Source: three-view drawing plus pictorial views. Frame: mm from the lowest corner of the part. A direction names the side the tool comes from. Give positions to 0.01 mm unless a question says otherwise; leave off trailing zeros. Order: outer loops, then holes, each group sorted by start corner. A loop starts at its lowest first (then second) coordinate and runs counter-clockwise, first axis right, second up. Notation, with made-up numbers: (-25.5, -15) -> (-3.5, -15) arc R36 cw to (-3.5, 22) -> close; hole circle Ø9 at (-26, 45.25). An arc over 180 degrees is marked (long way). Answer in a Markdown table with one row per item.
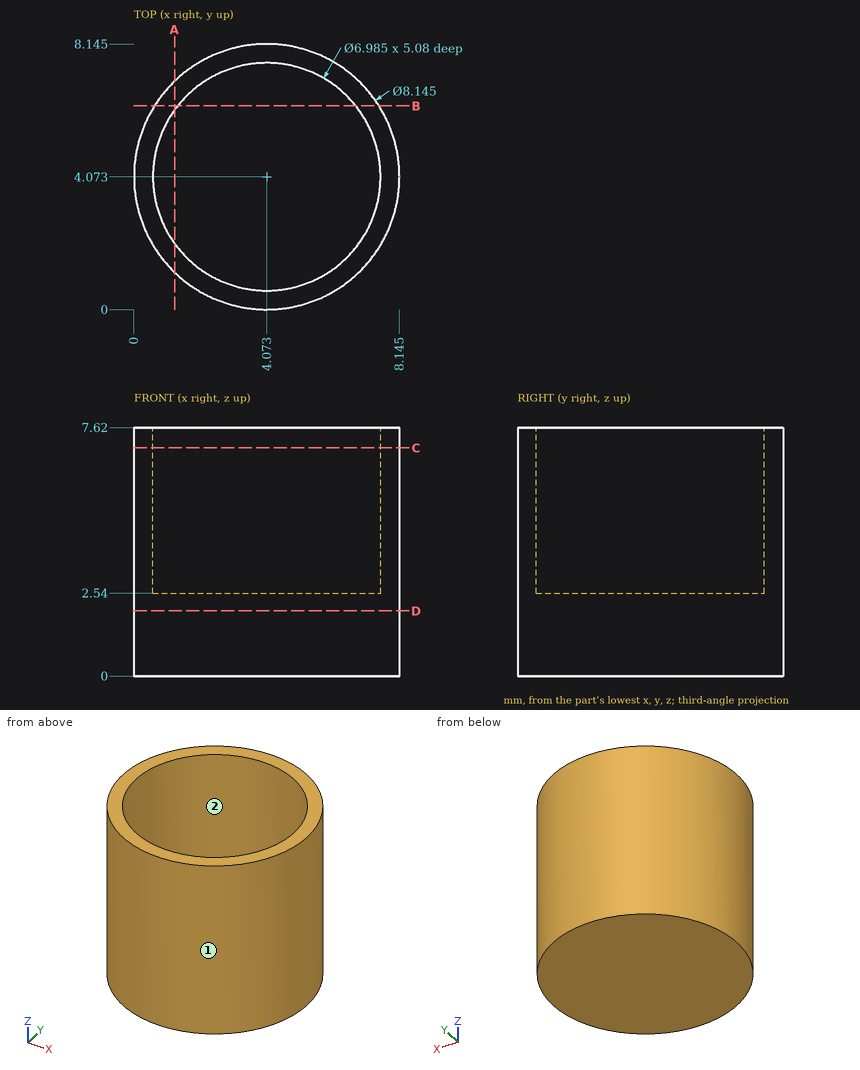
(1) Section query C-C (z = 7). Return the cut outline in (x, y) (1 decimal), plus the area to 3 significant figures.
A:
| item | result |
|---|---|
| outline | circle Ø8.1 at (4.1, 4.1); hole circle Ø7 at (4.1, 4.1) |
| area | 13.8 mm^2 |
(2) Section query A-A (x = 1.25). Return the cut outline in (y, z).
A:
| item | result |
|---|---|
| outline | (1.14, 0) -> (7.01, 0) -> (7.01, 7.62) -> (6.13, 7.62) -> (6.13, 2.54) -> (2.02, 2.54) -> (2.02, 7.62) -> (1.14, 7.62) -> close |
(3) Section query D-D (z = 2). Return the cut outline in (x, y) (1 decimal), plus the area to 3 significant figures.
A:
| item | result |
|---|---|
| outline | circle Ø8.1 at (4.1, 4.1) |
| area | 52.1 mm^2 |
(4) Ray query, probe 1 along Z at (x, y) = (2.75, 4); probe 2 along X at (y, z) = (5.25, 7) (1 decimal); probe 3 along Y at (x, z) = (1.25, 3.25) (1 decimal). Return the intervals inside material, ascending.
A:
| item | result |
|---|---|
| probe 1 | z = 0 to 2.54 |
| probe 2 | x = 0.2 to 0.8, 7.4 to 8 |
| probe 3 | y = 1.1 to 2, 6.1 to 7 |
(5) Access query for the marked faces 1 and 2. Directions: +Z, -Z, +X, -X, +Y, -Y. A direction counts if a zero-diameter tool reaches every point of the face in a straight line with its end or side. Return the directions, or none.
A:
| item | result |
|---|---|
| face 1 | +Z, -Z |
| face 2 | +Z |
(6) Section query B-B (y = 6.25). Return the cut outline in (x, z) (1 decimal).
A:
| item | result |
|---|---|
| outline | (0.6, 0) -> (7.5, 0) -> (7.5, 7.6) -> (6.8, 7.6) -> (6.8, 2.5) -> (1.3, 2.5) -> (1.3, 7.6) -> (0.6, 7.6) -> close |
(7) First-contact query: pin 1 Ø4 at (x, y) = (4, 3.5) entering from +Z. Flat tip, straight axial feed; report the tip coordinate or a pass-through.
A:
| item | result |
|---|---|
| pin 1 | stops at z = 2.54 |
